Autodesk Inventor part; units mm, degrees
ref_plane "YZ Plane" through (0, 0, 0) normal (1, 0, 0) x (0, 1, 0)
ref_plane "XZ Plane" through (0, 0, 0) normal (0, 1, 0) x (-1, 0, 0)
ref_plane "XY Plane" through (0, 0, 0) normal (0, 0, 1) x (1, 0, 0)
sketch "Sketch1" plane through (0, 0, 0) normal (0, 1, 0) x (-1, 0, 0)
  circle A0 centre (0, 0) radius 45
  dimension "d0" = 90
extrude "Extrusion1" add sketch "Sketch1" along normal blind 3
sketch "Sketch2" plane through (0, 3, 0) normal (0, 1, 0) x (1, 0, 0)
  circle A0 centre (0, 0) radius 45
  circle A1 centre (0, 0) radius 42.5
  circle A2 centre (0, 0) radius 43.25
  circle A3 centre (0, 0) radius 41.75
  dimension "d3" = 2.5
  dimension "d4" = 0.75
  dimension "d5" = 0.75
extrude "Extrusion2" cut sketch "Sketch2" against normal blind 2 contours A3
extrude "Extrusion3" cut sketch "Sketch2" against normal blind 2 contours A2
sketch "Sketch3" plane through (0, 1, 0) normal (0, 1, 0) x (1, 0, 0)
  circle A0 centre (0, 0) radius 40 construction
  line L0 (-40, 0) -> (40, 0) construction
  line L1 (0, 40) -> (0, -40) construction
  circle A1 centre (0, 35) radius 1.5
  circle A2 centre (35, 0) radius 1.5
  circle A3 centre (0, -35) radius 1.5
  circle A4 centre (0, 35) radius 4
  circle A5 centre (35, 0) radius 4
  circle A6 centre (0, -35) radius 4
  dimension "d10" = 80
  dimension "d12" = 3
  dimension "d13" = 3
  dimension "d14" = 5
  dimension "d15" = 5
  dimension "d17" = 3
  dimension "d18" = 5
  dimension "d19" = 2.5
  dimension "d20" = 2.5
  dimension "d21" = 2.5
extrude "Extrusion4" add sketch "Sketch3" along normal blind 0.75
extrude "Extrusion6" add sketch "Sketch3" along normal blind 4 contours A1 | A2 | A3
sketch "Sketch5" plane through (35, 5, 0) normal (0, 1, 0) x (1, 0, 0)
  circle A0 centre (0, 0) radius 4
  circle A1 centre (-35, -35) radius 4
  circle A2 centre (-35, 35) radius 4
  circle A3 centre (-35, 35) radius 1.5
  circle A4 centre (-35, 35) radius 1
  circle A5 centre (0, 0) radius 1.5
  circle A6 centre (0, 0) radius 1
  circle A7 centre (-35, -35) radius 1.5
  circle A8 centre (-35, -35) radius 1
  point P0 (-35, 0)
  dimension "d30" = 0.5
  dimension "d31" = 0.5
  dimension "d32" = 0.5
extrude "Extrusion7" cut sketch "Sketch5" against normal through all contours A4 | A6 | A8
properties part number "ROUNDBOTTOMCOVER"
The listing builds one solid part. Answer for the finished solid, in the listing's coordinates (mm). A direction names the side the tool comes from. Round coordinates to 2 decimals unless told otherwise and drop trailing zeros. Loops run counter-clockwise (first coordinate to the right, second up) from the corner with the lowest first, then second, coordinate; pieces in that order, holes last. Notation, with made-up numbers: M -15,26 L -2,26 A26 cw -2,52 Z; hole C 29.25,-5.75 d9. An arc over 180 degrees is marked long. Return JSON: item names as keys, results as strings.
Q1. Each of these flat-tipped pins is pushed along its axis until it touches: pin 1 Ø3 at (y, z) = (3.5, -29.5) entering from -X; pin 2 Ø1.5 at (y, z) = (3, 30) entering from +X; pin 3 Ø3 at (x, z) = (-12, -26.5) entering from +Y. Where does it stop, or does it pass through?
Results list:
{"pin 1": "stops at x = -35.16", "pin 2": "stops at x = 34.2", "pin 3": "stops at y = 1"}
Q2. Find the intervals of material crossed by line 1 along Z through (x, y) = (0, 3.3); line 2 along Z through (x, y) = (11, 2); line 3 along X through (y, z) = (1.4, -35), in increasing order. Write a range as from..to.
Results list:
{"line 1": "z = -36.5..-36, -34..-33.5, 33.5..34, 36..36.5", "line 2": "z = -43.63..-41.83, -41.05..-40.27, 40.27..41.05, 41.83..43.63", "line 3": "x = -28.28..-25.41, -24.11..-22.76, -4..-1, 1..4, 22.76..24.11, 25.41..28.28"}
Q3. Find section C-C, the plane z = -19.5. Determine the outline of the cut face in (x, y), plus the area to 3 significant figures.
Results list:
{"outline": "M -40.56,0 L 40.56,0 L 40.56,3 L 38.6,3 L 38.6,1 L 37.76,1 L 37.76,3 L 36.92,3 L 36.92,1 L -36.92,1 L -36.92,3 L -37.76,3 L -37.76,1 L -38.6,1 L -38.6,3 L -40.56,3 Z", "area": "92.3 mm2"}
Q4. Which of the six approach directions +Z, -Z, +X, -X, +Y, -Y give full straight-line access (tool end or side, diameter ignored) to faces 1 (the face through (0, 3, 34)), 2 (the face through (-1, 1, -1))?
Results list:
{"face 1": "+Y, -Y", "face 2": "+Y"}
Q5. Find section B-B, the plane x = 10. Determine the outline of the cut face in (y, z), plus the area to 3 significant figures.
Results list:
{"outline": "M 0,-43.87 L 3,-43.87 L 3,-42.08 L 1,-42.08 L 1,-41.31 L 3,-41.31 L 3,-40.53 L 1,-40.53 L 1,40.53 L 3,40.53 L 3,41.31 L 1,41.31 L 1,42.08 L 3,42.08 L 3,43.87 L 0,43.87 Z", "area": "98.0 mm2"}
Q6. Find section A-A, the plane y = 4. Determine the outline of the cut face in (x, z).
Results list:
{"outline": "C 0,-35 d3; C 0,35 d3; C 35,0 d3; hole C 0,-35 d2; hole C 0,35 d2; hole C 35,0 d2"}
Q7. The mould has two halves that part along Z. Classify faces 3 (the face through (-20.765, 1.479, 39.923)), 4 (the face through (31.8, 1.4, -2.4)), 5 (the face through (37, 1.75, 0)), 6 (the face through (1, 0, 1)): released by +Z, released by -Z, zero draft, split by the parting line, or undercut.
Results list:
{"face 3": "split by the parting line", "face 4": "undercut", "face 5": "undercut", "face 6": "zero draft"}
